Could you check a few things on this model? Use its own coordinates, in mm. A direction names the side the tool comes from. Coordinates: 2 decimals unless noted, no trailing zeros. Loops run counter-clockwise (first coordinate to the right, second up) from the corner with the lowest first, then second, coordinate; pieces in that order, holes last. Notation, with made-up numbers: (-38.5, 68) -> (4.5, 68) arc R34 ccw to (4.5, 106) -> close; hole circle Ø4 at (69, 87). An arc over 180 degrees is marked (long way). One line per question, with ' | ' between items. Start each with the question number.
(1) Suppose I cut it at D-D (x = -6.25). Please give me the cut outline in (y, z).
(2) Suppose I cut it at B-B (y = -2.54). Please give me the cut outline in (x, z) (3 decimals).
(3) Suppose I cut it at A-A (x = 5.08). Please give me the cut outline in (y, z) (3 decimals).
(4) Which directions (+Z, -Z, +X, -X, +Y, -Y) give clear straight access to the entire face, cutting with the end or side of a thin tool? Please do faces 1 (the face through (1.2, 0, 2)), 2 (the face through (0, -2, 0)).
(5) If I drill on line 1 along Y through (x, z) = (5.08, 0.95) (3 decimals); line 2 along X through (y, z) = (-4, 1.55); line 3 along X through (y, z) = (-2.25, 0.7), over which ranges is the centre line in solid material (lowest first)?
(6) If we mould it in two halves opening along X, with no side actions, what happens to faces 3 (the face through (-7.62, -2, 1)), 4 (the face through (0, -2, 1.702)), 5 (the face through (-3.263, -1.968, 0.863))? For each: pulls with the +X half, pulls with the -X half, needs draft (parallel to the pull), parting line crosses it, or undercut.
(7) Suppose I cut it at C-C (z = 1.3). Please give me the cut outline in (x, y) (3 decimals), plus the area to 3 significant figures.
(8) I'm going to push flat-ended pins straight in: pin 1 Ø4 at (x, y) = (-4, -1.5) entering from +Z; pin 2 Ø6 at (x, y) = (5.5, -5) entering from -Z; pin 3 Ø0.6 at (x, z) = (-0.5, 2.5) entering from +Y; pin 4 Ø0.6 at (x, z) = (0, 2.5) entering from -Y. Where does each tip first touch, or does it pass through?
Autodesk Inventor part; units mm, degrees
ref_plane "YZ Plane" through (0, 0, 0) normal (1, 0, 0) x (0, 1, 0)
ref_plane "XZ Plane" through (0, 0, 0) normal (0, 1, 0) x (-1, 0, 0)
ref_plane "XY Plane" through (0, 0, 0) normal (0, 0, 1) x (1, 0, 0)
sketch "Sketch1" plane through (0, 0, 0) normal (0, 0, 1) x (1, 0, 0)
  line L0 (-7.62, -7.62) -> (7.62, -7.62)
  line L1 (7.62, -7.62) -> (7.62, 2.54)
  line L2 (7.62, 2.54) -> (-7.62, 2.54)
  line L3 (-7.62, 2.54) -> (-7.62, -7.62)
  line L4 (-10.668, 0) -> (10.668, 0) construction
  line L5 (0, -9.652) -> (0, 4.572) construction
  point P0 (0, 0)
  dimension "d0" = 10.16
  dimension "d1" = 15.24
  dimension "d2" = 2.54
extrude "Extrusion1" add sketch "Sketch1" along normal blind 1.7018
sketch "Sketch2" plane through (0, 0, 1.7018) normal (0, 0, 1) x (1, 0, 0)
  line L0 (-7.62, -7.62) -> (-7.62, 2.54)
  line L1 (7.62, -7.62) -> (-7.62, -7.62)
  line L2 (7.62, 2.54) -> (7.62, -7.62)
  line L3 (-7.62, 2.54) -> (7.62, 2.54)
  line L4 (-10.668, 0) -> (10.668, 0) construction
  line L5 (0, -9.652) -> (0, 4.572) construction
  line L6 (-7.62, -2.54) -> (7.62, -2.54) construction
  circle A0 centre (-5.08, -2.54) radius 1.905
  circle A1 centre (5.08, -2.54) radius 1.905
  point P0 (0, 0)
  dimension "d5" = 10.16
  dimension "d6" = 3.81
extrude "Extrusion2" cut sketch "Sketch2" against normal through all contours A0 | A1
sketch "Sketch3" plane through (0, 0, 1.7018) normal (0, 0, 1) x (1, 0, 0)
  line L0 (-10.668, 0) -> (10.668, 0) construction
  line L1 (0, -9.652) -> (0, 4.572) construction
  line L2 (-1.2001, 0.4) -> (1.2002, 0.4001)
  line L3 (1.2002, 0.4001) -> (1.2002, -0.4001)
  line L4 (1.2002, -0.4001) -> (-1.2001, -0.4)
  line L5 (-1.2001, -0.4) -> (-1.2001, 0.4)
  point P0 (0, 0)
  dimension "d9" = 0.8001
  dimension "d10" = 2.4003
extrude "Extrusion3" add sketch "Sketch3" along normal blind 1.27
sketch "Sketch4" plane through (0, 0, 0) normal (0, 0, -1) x (-1, 0, 0)
  circle A0 centre (2.54, 0.1778) radius 0.635
  circle A1 centre (0, 0.1778) radius 0.635
  circle A2 centre (-2.54, 0.1778) radius 0.635
  point P0 (0, 0)
properties part number "J002609"
Checks:
1) outline: (-7.62, 0) -> (-4.04, 0) -> (-4.04, 1.7) -> (-7.62, 1.7) -> close; (-1.04, 0) -> (2.54, 0) -> (2.54, 1.7) -> (-1.04, 1.7) -> close
2) outline: (-7.62, 0) -> (-6.985, 0) -> (-6.985, 1.702) -> (-7.62, 1.702) -> close; (-3.175, 0) -> (3.175, 0) -> (3.175, 1.702) -> (-3.175, 1.702) -> close; (6.985, 0) -> (7.62, 0) -> (7.62, 1.702) -> (6.985, 1.702) -> close
3) outline: (-7.62, 0) -> (-4.445, 0) -> (-4.445, 1.702) -> (-7.62, 1.702) -> close; (-0.635, 0) -> (2.54, 0) -> (2.54, 1.702) -> (-0.635, 1.702) -> close
4) face 1: +Z, +X, +Y, -Y | face 2: -Z, +X, -X, +Y, -Y
5) line 1: y = -7.62 to -4.445, -0.635 to 2.54 | line 2: x = -7.62 to -6.3, -3.86 to 3.86, 6.3 to 7.62 | line 3: x = -7.62 to -6.96, -3.2 to 3.2, 6.96 to 7.62
6) face 3: pulls with the -X half | face 4: needs draft | face 5: undercut
7) outline: (-7.62, -7.62) -> (7.62, -7.62) -> (7.62, 2.54) -> (-7.62, 2.54) -> close; hole circle Ø3.81 at (-5.08, -2.54); hole circle Ø3.81 at (5.08, -2.54) | area: 132 mm^2
8) pin 1: stops at z = 1.7 | pin 2: stops at z = 0 | pin 3: stops at y = 0.4 | pin 4: stops at y = -0.4
